from build123d import *

# Parameters (mm, degrees)
SKETCH1_R           = 4
SKETCH1_R_2         = 3
SKETCH1_R_3         = 6
SKETCH1_R_4         = 5
BOSS_EXTRUDE1_DEPTH = 2
SKETCH1_3_R         = 5
BOSS_EXTRUDE2_DEPTH = 3
BOSS_EXTRUDE3_START = -2
SKETCH1_4_R         = 3
BOSS_EXTRUDE3_DEPTH = 12


with BuildPart() as part:
    # Sketch1 → Boss-Extrude1 (new, symmetric)
    # profile 1 of 3: a face of its own
    with BuildSketch(Plane.YZ):
        with BuildLine():
            ThreePointArc((-8.18, 29.08), (-12.18, 25.08), (-16.18, 29.08))
            Line((-16.18, 29.08), (-16.18, 4.569972731))
            Line((-16.18, 4.569972731), (-3.584071428, -4.811905236))
            ThreePointArc((-3.584071428, -4.811905236), (-5.998168777, 0.148227284), (-3.342017287, 4.98306336))
            Line((-3.342017287, 4.98306336), (-8.18, 8.586558185))
            Line((-8.18, 8.586558185), (-8.18, 29.08))
        make_face()
    # profile 2 of 3: a face of its own
    with BuildSketch(Plane.YZ):
        with Locations((-12.18, 29.08)):
            Circle(SKETCH1_R)
        with Locations(Location((-12.18, 29.08, 0), (0, 0, 270))):
            Circle(SKETCH1_R_2, mode=Mode.SUBTRACT)
    # profile 3 of 3: a face of its own
    with BuildSketch(Plane.YZ):
        Circle(SKETCH1_R_3)
        with Locations(Location((0, 0, 0), (0, 0, 270))):
            Circle(SKETCH1_R_4, mode=Mode.SUBTRACT)
    extrude(amount=BOSS_EXTRUDE1_DEPTH, both=True)

    # Sketch1<3> → Boss-Extrude2 (add, symmetric)
    with BuildSketch(Plane.YZ):
        with Locations(Location((0, 0, 0), (0, 0, 270))):
            Circle(SKETCH1_3_R)
    extrude(amount=BOSS_EXTRUDE2_DEPTH, both=True)

    # Sketch1<4> → Boss-Extrude3 (add)
    with BuildSketch(Plane.YZ.offset(BOSS_EXTRUDE3_START)):
        with Locations(Location((-12.18, 29.08, 0), (0, 0, 270))):
            Circle(SKETCH1_4_R)
    extrude(amount=BOSS_EXTRUDE3_DEPTH)


solid = part.part
Design review of the part built by this model. Coordinates are the model's own, in mm. A direction names the side the tool comes from. Coordinates: 2 decimals unless noted, no trailing zeros. Loops run counter-clockwise (first coordinate to the right, second up) from the corner with the lowest first, then second, coordinate; pieces in that order, holes last.
Item 1: Add section C-C (z = 0). Write out the cut boundary in (x, y).
Completed:
outline: (-3, -5) - (-2, -5) - (-2, -10.04) - (2, -10.04) - (2, -5) - (3, -5) - (3, 5) - (2, 5) - (2, 6) - (-2, 6) - (-2, 5) - (-3, 5) - close
Item 2: Add section D-D (y = -13). Write out the cut boundary in (x, z).
Completed:
outline: (-2, 2.2) - (2, 2.2) - (2, 26.19) - (10, 26.19) - (10, 31.97) - (2, 31.97) - (2, 33) - (-2, 33) - close
Item 3: Add section B-B (y = 0). Write out the cut boundary in (x, z).
Completed:
outline: (-3, -5) - (-2, -5) - (-2, -6) - (2, -6) - (2, -5) - (3, -5) - (3, 5) - (2, 5) - (2, 6) - (-2, 6) - (-2, 5) - (-3, 5) - close
Item 4: Clearance check with flat-ended pins moving along their axes: pin 1 (6.5 mm diameter, centred on y = -13.5, z = 30, fed in from -X); pin 2 (1.2 mm diameter, centred on x = -0.5, z = 17.5, fed in from +Y); pin 3 (3 mm diameter, centred on y = -2, z = 0, fed in from +X). State where each tip first meets the part, or that it passes through.
Completed:
pin 1: stops at x = -2
pin 2: stops at y = -8.18
pin 3: stops at x = 3
Item 5: Wall thickness on L1, parallel to X at y = -2, z = 4.5; L2, parallel to X at y = -11.75, z = 19; L3, parallel to Z at x = 3, y = -11.5: over which ranges is each line inside the solid? List them lowest first.
Completed:
L1: x = -3 to 3
L2: x = -2 to 2
L3: z = 26.16 to 32
Item 6: Draft analysis for pull direction Y (two halves, no side actions). For faces 1 (the flat face through (10, -12, 29)), 2 (the cylindrical face through (2.51, -4.88, 1.08)), 3 (the flat face through (0.03, -5.73, 6.76)), 4 (the flat face through (0, -8.18, 19)), state which applies: pulls with the +Y half, pulls with the -Y half, needs draft (parallel to the pull), parting line crosses it, or undercut.
Completed:
face 1: needs draft
face 2: parting line crosses it
face 3: undercut
face 4: pulls with the +Y half
Item 7: For faces 5 (the cylindrical face through (-2.49, -4.88, 1.08)), 6 (the cylindrical face through (5.944, -12.048, 32.077)), 7 (the flat face through (-3, 0, 0)), list the 3-axis set-ups (+Z, -Z, +X, -X, +Y, -Y) from which the entire face can be reached by the end or side of a thin tool; tool diameter is ignored.
Completed:
face 5: -X
face 6: +X
face 7: +Z, -Z, -X, +Y, -Y
Item 8: Add section A-A (x = 1.5). Write out the cut boundary in (y, z).
Completed:
outline: (-16.18, 4.57) - (-3.58, -4.81) arc R6 ccw (long way) to (-3.34, 4.98) - (-8.18, 8.59) - (-8.18, 29.08) arc R4 ccw to (-16.18, 29.08) - close
